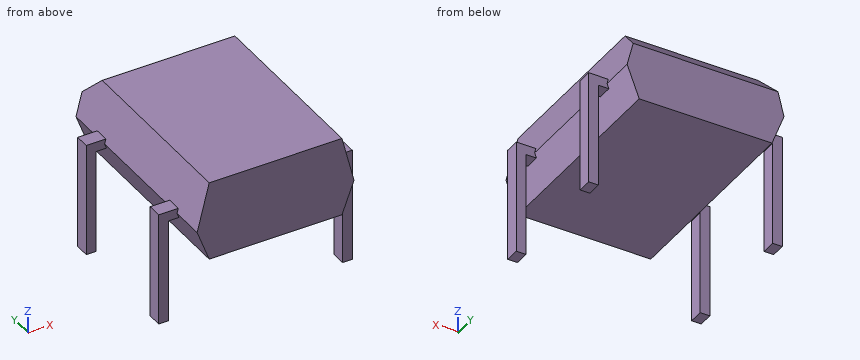
from build123d import *

# Parameters (mm, degrees)
PAD002_DEPTH = 0.3
PAD_DEPTH    = 4.25
CHAMFER_SIZE = 0.99
PAD001_DEPTH = 0.3


with BuildPart() as pad002:
    # Sketch002 → Pad002 (new body, symmetric)
    with BuildSketch(Plane.XZ.offset(5.08)):
        Polygon((-0.2, -3), (0.2, -3), (0.2, 1.32), (7.42, 1.32), (7.42, -3), (7.82, -3), (7.82, 1.72), (-0.2, 1.72), align=None)
    extrude(amount=PAD002_DEPTH, both=True)


with BuildPart() as chamfer_body:
    # Sketch → Pad (new body, symmetric)
    with BuildSketch(Plane.XZ.offset(2.54)):
        Polygon((1.06, 0.2), (6.56, 0.2), (7.06, 1.52), (6.56, 3.5), (1.06, 3.5), (0.56, 1.52), align=None)
    extrude(amount=PAD_DEPTH, both=True)

    # Chamfer
    chamfer_edges = [chamfer_body.edges().sort_by_distance(p)[0] for p in [
        (3.81, 1.71, 3.5),
    ]]
    chamfer(chamfer_edges, length=CHAMFER_SIZE)


with BuildPart() as diode_bridge_dip_4_w7_62mm_p5_08mm:
    # Sketch001 → Pad001 (new body, symmetric)
    with BuildSketch(Plane.XZ):
        Polygon((-0.2, -3), (0.2, -3), (0.2, 1.32), (7.42, 1.32), (7.42, -3), (7.82, -3), (7.82, 1.72), (-0.2, 1.72), align=None)
    extrude(amount=PAD001_DEPTH, both=True)

    add(pad002.part)
    add(chamfer_body.part)


solid = diode_bridge_dip_4_w7_62mm_p5_08mm.part
Verification items for the finished model (mm, model axes). Round coordinates to 2 decimals unless told otherwise and drop trailing zeros. Loops run counter-clockwise (first coordinate to the right, second up) from the corner with the lowest first, then second, coordinate; pieces in that order, holes last. Notation, with made-up numbers: M -17,6 L 12,6 A26 cw 12,40 Z; hole C 12.25,88 d11. An arc over 180 degrees is marked long. Write each question's results on one line, items separated by ' | '.
1) Gauge pin test, flat ends, axial feed: P1, Ø0.7, axis at x = 7.5, y = 0, coming from the +Z side; P2, Ø1.6, axis at x = 3, y = -2, coming from the -Z side. Record the tip position at first contact, or that the pin passes through.
Checks:
P1: stops at z = 1.72 | P2: stops at z = 0.2
2) Section check B-B on z = -2.5. Record the boundary of the cut face in (x, y).
Checks:
outline: M -0.2,-5.38 L 0.2,-5.38 L 0.2,-4.78 L -0.2,-4.78 Z; M -0.2,-0.3 L 0.2,-0.3 L 0.2,0.3 L -0.2,0.3 Z; M 7.42,-5.38 L 7.82,-5.38 L 7.82,-4.78 L 7.42,-4.78 Z; M 7.42,-0.3 L 7.82,-0.3 L 7.82,0.3 L 7.42,0.3 Z
3) Section check D-D on x = 1.25. Record the boundary of the cut face in (y, z).
Checks:
outline: M -6.79,0.2 L 1.71,0.2 L 1.71,2.51 L 0.72,3.5 L -6.79,3.5 Z
4) Section check C-C on y = -5. Record the boundary of the cut face in (x, z), then the cut area to 3 significant figures.
Checks:
outline: M -0.2,-3 L 0.2,-3 L 0.2,1.32 L 0.64,1.32 L 1.06,0.2 L 6.56,0.2 L 6.98,1.32 L 7.42,1.32 L 7.42,-3 L 7.82,-3 L 7.82,1.72 L 7.01,1.72 L 6.56,3.5 L 1.06,3.5 L 0.61,1.72 L -0.2,1.72 Z | area: 23.9 mm2
5) Scan lines: L1, parallel to X at y = 0.25, z = -1.5; L2, parallel to Z at x = 3, y = -4.75; L3, parallel to Y at x = 3.75, z = 3. Record each from-to range of solid material in increasing order. Write a range as from..to.
Checks:
L1: x = -0.2..0.2, 7.42..7.82 | L2: z = 0.2..3.5 | L3: y = -6.79..1.22
6) Section check A-A on x = 7.25. Record the boundary of the cut face in (y, z).
Checks:
outline: M -5.38,1.32 L -4.78,1.32 L -4.78,1.72 L -5.38,1.72 Z; M -0.3,1.32 L 0.3,1.32 L 0.3,1.72 L -0.3,1.72 Z
